from build123d import *

# Parameters (mm, degrees)
F1_DEPTH = 4.572


with BuildPart() as f1:
    # F0 (on Top) → F1 (new body)
    with BuildSketch(Plane.XY):
        with BuildLine():
            ThreePointArc((-6.593841, 49.071565), (-30.72384, 53.027217), (-54.85384, 49.071565))
            Line((-54.85384, 49.071565), (-54.85384, 38.911565))
            Line((-54.85384, 38.911565), (-48.50384, 38.911565))
            Line((-48.50384, 38.911565), (-48.50384, 19.861565))
            Line((-48.50384, 19.861565), (-54.85384, 19.861565))
            Line((-54.85384, 19.861565), (-54.85384, -25.858435))
            Line((-54.85384, -25.858435), (-48.50384, -25.858435))
            Line((-48.50384, -25.858435), (-48.50384, -44.908435))
            Line((-48.50384, -44.908435), (-54.85384, -44.908435))
            Line((-54.85384, -44.908435), (-54.85384, -52.528435))
            ThreePointArc((-54.85384, -52.528435), (-30.72384, -60.853284), (-6.593841, -52.528435))
            Line((-6.593841, -52.528435), (-6.593841, -44.908435))
            Line((-6.593841, -44.908435), (-12.943841, -44.908435))
            Line((-12.943841, -44.908435), (-12.943841, -25.858435))
            Line((-12.943841, -25.858435), (-6.593841, -25.858435))
            Line((-6.593841, -25.858435), (-6.593841, 19.861565))
            Line((-6.593841, 19.861565), (-12.943841, 19.861565))
            Line((-12.943841, 19.861565), (-12.943841, 38.911565))
            Line((-12.943841, 38.911565), (-6.593841, 38.911565))
            Line((-6.593841, 38.911565), (-6.593841, 49.071565))
        make_face()
    extrude(amount=F1_DEPTH)


solid = f1.part
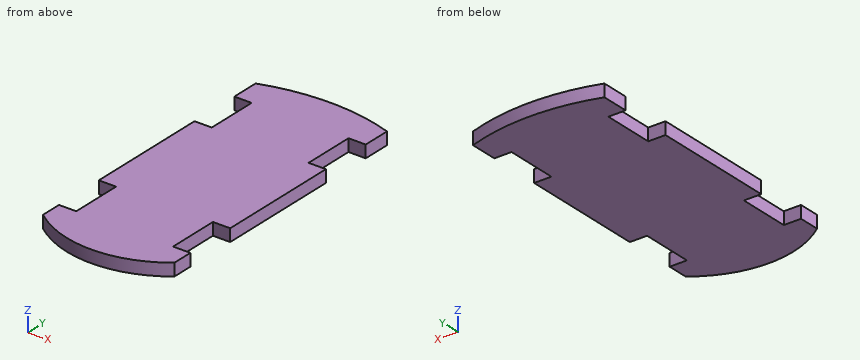
The listing builds one solid part. Answer for the finished solid, in the listing's coordinates (mm). Give positions to 0.01 mm unless a question says otherwise; leave off trailing zeros. Write each loop counter-clockwise with the first axis right and the second up, starting at its lowest first coordinate (ties: lowest second). Pieces come first, ordered by that corner, then holes.
Item 1: Section B-B, the plane x = -10 is taken. Write down the section's boundary in (y, z), plus the area to 3 significant figures.
Item 2: Section D-D, the plane x = -17 is taken. Write down the section's boundary in (y, z), plus the area to 3 significant figures.
Item 3: Flat-ended cylindrical pins translate along their axes: P1, Ø2.5, axis at y = -32.5, z = 3.5, coming from the +X side; P2, Ø2.5, axis at x = -9, z = 2.5, coming from the -Y side; P3, Ø1.4, axis at x = -50.5, z = 2.5, coming from the -Y side. Find the tip coordinate at first contact, or state that the pin passes through.
Item 4: Find the intervals of material crossed by line 1 along Y through (x, z) = (-31.5, 2.9); line 2 along X through (y, z) = (-32, 2.45); line 3 along Y through (x, z) = (-51, 0.35), in increasing order.
Item 5: Section C-C, the plane y = 26.5 is taken. Write down the section's boundary in (x, z).
Item 6: Section A-A, the plane z = 1.35 is taken. Write down the section's boundary in (x, y), plus the area to 3 significant figures.
Completed:
1. outline: (-54.92, 0) - (-44.91, 0) - (-44.91, 4.57) - (-54.92, 4.57) - close; (-25.86, 0) - (19.86, 0) - (19.86, 4.57) - (-25.86, 4.57) - close; (38.91, 0) - (50.13, 0) - (50.13, 4.57) - (38.91, 4.57) - close
1. area: 306 mm2
2. outline: (-58.37, 0) - (51.77, 0) - (51.77, 4.57) - (-58.37, 4.57) - close
2. area: 504 mm2
3. P1: stops at x = -12.94
3. P2: stops at y = -55.07
3. P3: stops at y = -55.89
4. line 1: y = -60.85 to 53.02
4. line 2: x = -48.5 to -12.94
4. line 3: y = -55.19 to -44.91, -25.86 to 19.86, 38.91 to 50.26
5. outline: (-48.5, 0) - (-12.94, 0) - (-12.94, 4.57) - (-48.5, 4.57) - close
6. outline: (-54.85, -52.53) arc R39.13 ccw to (-6.59, -52.53) - (-6.59, -44.91) - (-12.94, -44.91) - (-12.94, -25.86) - (-6.59, -25.86) - (-6.59, 19.86) - (-12.94, 19.86) - (-12.94, 38.91) - (-6.59, 38.91) - (-6.59, 49.07) arc R75.58 ccw to (-54.85, 49.07) - (-54.85, 38.91) - (-48.5, 38.91) - (-48.5, 19.86) - (-54.85, 19.86) - (-54.85, -25.86) - (-48.5, -25.86) - (-48.5, -44.91) - (-54.85, -44.91) - close
6. area: 4,820 mm2
